Verification items for this drawing (mm, ordinates from the low corner). A direction names the side the tool comes from. Round coordinates to 2 decimals unless told otherwise and drop trailing zeros. Loops run counter-clockwise (first coordinate to the right, second up) from the corner with the lowest first, then second, coordinate; pieces in that order, holes last. Notation, with made-up numbers: (-28.5, 73) -> (23.5, 73) arc R17 ccw to (23.5, 82) -> close; hole circle Ø1 at (70, 69.5). An arc over 180 degrees is marked (long way). One line per question, with ' | ' between items.
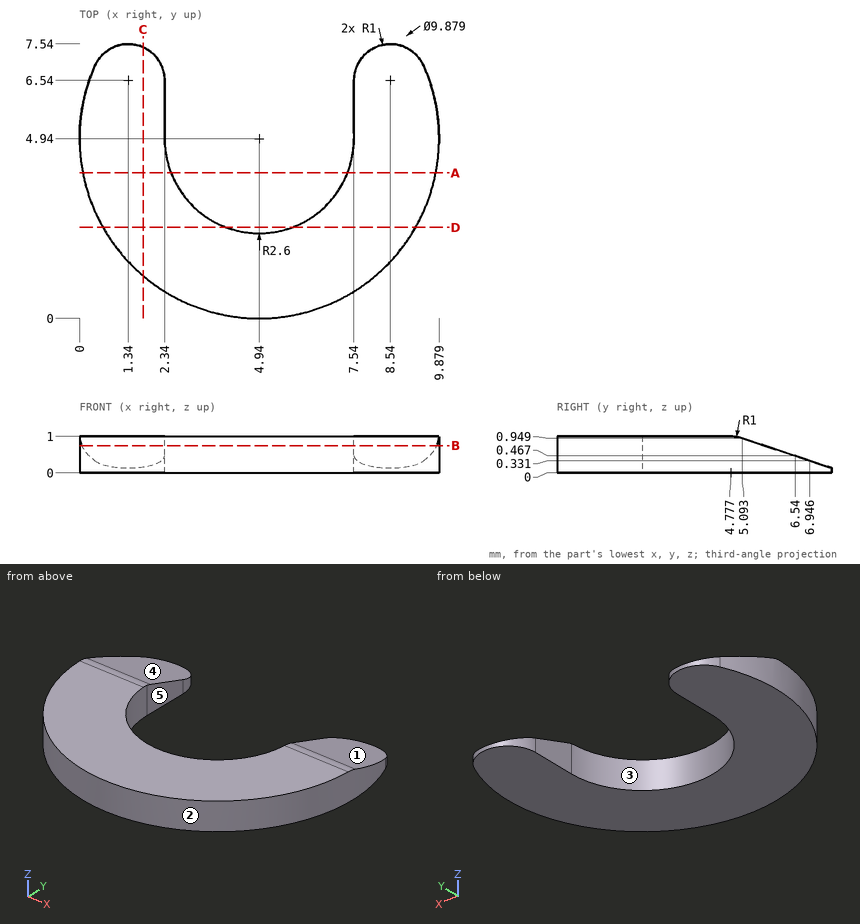
(1) Sectioned sample at B-B, the plane z = 0.75. Record the cut outline in (x, y), and give its area (3 significant figures).
Answer:
outline: (0.06, 5.69) arc R4.94 ccw (long way) to (9.82, 5.69) -> (7.54, 5.69) -> (7.54, 4.94) arc R2.6 cw to (2.34, 4.94) -> (2.34, 5.69) -> close | area: 31.2 mm2
(2) Go/stop test with flat-tipped pins: pin 1 (0.5 mm diameter, centred on y = 5.5, z = 0.5, fed in from +X); pin 2 (2 mm diameter, centred on x = 5, y = 5.5, fed in from +Z); pin 3 (0.5 mm diameter, centred on y = 5.5, z = 0.5, fed in from -X). Record where each tip stops, or that it passes through.
Answer:
pin 1: stops at x = 9.87 | pin 2: passes through | pin 3: stops at x = 0.01
(3) Sectioned sample at C-C, the plane x = 1.75. Record the cut outline in (y, z).
Answer:
outline: (1.17, 0) -> (7.45, 0) -> (7.45, 0.16) -> (5.09, 0.95) arc R1 ccw to (4.78, 1) -> (1.17, 1) -> close
(4) Sectioned sample at A-A, the plane y = 4. Record the cut outline in (x, z) (1 decimal).
Answer:
outline: (0.1, 0) -> (2.5, 0) -> (2.5, 1) -> (0.1, 1) -> close; (7.4, 0) -> (9.8, 0) -> (9.8, 1) -> (7.4, 1) -> close
(5) Sectioned sample at D-D, the plane y = 2.5. Record the cut outline in (x, z) (1 decimal).
Answer:
outline: (0.6, 0) -> (4, 0) -> (4, 1) -> (0.6, 1) -> close; (5.8, 0) -> (9.2, 0) -> (9.2, 1) -> (5.8, 1) -> close
(6) Scan lines: probe 1 along X at (y, z) = (4.75, 0.6) (1 decimal); probe 2 along Y at (x, z) = (5, 0.6); probe 3 along X at (y, z) = (1.5, 0.9) (1 decimal). Record each from-to range of solid material in increasing order.
Answer:
probe 1: x = 0 to 2.3, 7.5 to 9.9 | probe 2: y = 0 to 2.34 | probe 3: x = 1.4 to 8.5
(7) Set-up check for the marked faces 4 and 5: record each of +Z, -Z, +X, -X, +Y, -Y from which the full face is reachable in a straight line by a thin tool's end or side.
Answer:
face 4: +Z, +X, -X, +Y | face 5: +Z, -Z, +Y
(8) Mould release check, pull along X, two halves, no side actions. Record for the marked faces 1, 2 and 3: +X half, -X half, draft (parallel to the pull), parting line (faces both ways), or undercut.
Answer:
face 1: draft | face 2: parting line | face 3: undercut
